```python
from build123d import *

# Parameters (mm, degrees)
BOSS_EXTRUDE1_DEPTH = 11.25
SKETCH1_3_R         = 25
SKETCH1_3_R_2       = 15
BOSS_EXTRUDE2_DEPTH = 30
CUT_EXTRUDE1_START  = -30
SKETCH3_R           = 2.5
CUT_EXTRUDE1_DEPTH  = 31


with BuildPart() as part:
    # Sketch1 → Boss-Extrude1 (new body, symmetric)
    with BuildSketch(Plane.XY):
        with BuildLine():
            ThreePointArc((-80.369346148, -16.271699348), (0, 82), (80.369346148, -16.271699348))
            add(Edge.make_bspline(
                [(96.539745155, 0), (97.326558794, -29.331535138), (77.47349205, -47.573942744), (78.112479352, -27.418839229), (80.369346148, -16.271699348)],
                knots=[0, 0, 0, 0, 0.663724029, 1, 1, 1, 1], degree=3))
            add(Edge.make_bspline(
                [(96.539745155, 0), (96.493331921, 1.730233625), (104.346209231, 42.222860352), (25, 135.629553039), (25, 154)],
                knots=[0, 0, 0, 0, 0.598565743, 1, 1, 1, 1], degree=3))
            ThreePointArc((25, 154), (0, 129), (-25, 154))
            add(Edge.make_bspline(
                [(-96.539745155, 0), (-96.493331921, 1.730233625), (-104.346209231, 42.222860352), (-25, 135.629553039), (-25, 154)],
                knots=[0, 0, 0, 0, 0.598565743, 1, 1, 1, 1], degree=3))
            add(Edge.make_bspline(
                [(-96.539745155, 0), (-97.326558794, -29.331535138), (-77.47349205, -47.573942744), (-78.112479352, -27.418839229), (-80.369346148, -16.271699348)],
                knots=[0, 0, 0, 0, 0.663724029, 1, 1, 1, 1], degree=3))
        make_face()
    extrude(amount=BOSS_EXTRUDE1_DEPTH, both=True)

    # Sketch1<3> → Boss-Extrude2 (add, symmetric)
    with BuildSketch(Plane.XY):
        with Locations((0, 154)):
            Circle(SKETCH1_3_R)
        with Locations((0, 154)):
            Circle(SKETCH1_3_R_2, mode=Mode.SUBTRACT)
    extrude(amount=BOSS_EXTRUDE2_DEPTH, both=True)

    # Sketch3 → Cut-Extrude1 (cut, through all)
    with BuildSketch(Plane(origin=(0, 180, 0), x_dir=(1, 0, 0), z_dir=(0, 1, 0)).offset(CUT_EXTRUDE1_START)):
        Circle(SKETCH3_R)
    extrude(amount=CUT_EXTRUDE1_DEPTH, mode=Mode.SUBTRACT)


solid = part.part
```
Could you check a few things on this model? Use its own coordinates, in mm. A direction names the side the tool comes from. Give positions to 0.01 mm unless a question says otherwise; leave off trailing zeros. Write each loop counter-clockwise with the first axis right and the second up, starting at its lowest first coordinate (ties: lowest second). Pieces come first, ordered by that corner, then holes. Notation, with made-up numbers: (86, 39) - (98, 39) arc R36 ccw to (98, 77) - close; hole circle Ø5 at (-19.75, -19.75). An arc over 180 degrees is marked (long way). One line per item, written item: value. Start each with the question number.
Item 1: Imagine slicing it at C-C, the plane x = 20.5. List the corners of the cut face in (y, z) for me.
Item 2: I'm going to push flat-ended pins straight in: pin 1 (6 mm diameter, centred on x = 22, z = -3.5, fed in from +Y); pin 2 (1.5 mm diameter, centred on x = 34, z = 13, fed in from +Y); pin 3 (1 mm diameter, centred on x = -24.5, z = 0, fed in from -Y); pin 4 (8 mm diameter, centred on x = 0, z = 0, fed in from +Y). Where does each tip first touch, or does it pass through?
Item 3: Which directions (+Z, -Z, +X, -X, +Y, -Y) give clear straight access to the entire face, cutting with the end or side of a thin tool? Please do faces 4 (the face through (-2.032, 81.975, 0.158)), 5 (the face through (-3.255, 178.787, 0.42)).
Item 4: Imagine slicing it at B-B, the plane z = -15.5. List the corners of the cut face in (x, y) for me.
Item 5: If we mould it in two halves opening along Z, with no side actions, what happens to faces 1 (the face through (0, 84, 11.25)), 2 (the face through (0, 84, -11.25)), 3 (the face through (-0.54, 173.82, 2.44))? For each: +Z half, -Z half, draft (parallel to the pull), parting line (faces both ways), or undercut.
Item 6: Imagine slicing it at A-A, the plane x = 0. List the corners of the cut face in (y, z) for me.
Item 7: Please list where these lines run through material, in increasing order: line 1 (Y direction, x = 0, z = -3); line 2 (X direction, y = 0, z = 1.25); line 3 (Z direction, x = 0, y = 172.5). Write a range as from..to.
Geometry says:
1. outline: (79.4, -11.25) - (139.69, -11.25) - (139.69, -30) - (168.31, -30) - (168.31, 30) - (139.69, 30) - (139.69, 11.25) - (79.4, 11.25) - close
2. pin 1: y = 170.25
2. pin 2: through
2. pin 3: y = 78.1
2. pin 4: y = 179
3. face 4: +Z, -Z
3. face 5: none
4. outline: circle Ø50 at (0, 154); hole circle Ø30 at (0, 154)
5. face 1: +Z half
5. face 2: -Z half
5. face 3: undercut
6. outline: (82, -11.25) - (129, -11.25) - (129, -30) - (139, -30) - (139, 30) - (129, 30) - (129, 11.25) - (82, 11.25) - close; (169, -30) - (179, -30) - (179, -2.5) - (169, -2.5) - close; (169, 2.5) - (179, 2.5) - (179, 30) - (169, 30) - close
7. line 1: 82..139, 169..179
7. line 2: -96.54..-82, 82..96.54
7. line 3: -30..-2.5, 2.5..30
